Here's how the part is built. I have some questions about the finished solid (model axes, mm). Give positions to 0.01 mm unless a question says otherwise; leave off trailing zeros. Loops run counter-clockwise (first coordinate to the right, second up) from the corner with the lowest first, then second, coordinate; pieces in that order, holes last.
Q1. If we section it at C-C (x = -3): Please give me the cut outline in (y, z).
Q2. If we section it at A-A (z = 0): Please give me the cut outline in (x, y) (3 decimals), plus the area to 4 significant figures.
Q3. I need wall thicknesses on line 1 (X direction, y = 2, z = 0) (3 decimals); line 2 (X direction, y = -0.5, z = 1.75) (3 decimals); line 3 (Z direction, x = -3.5, y = 2). Which ranges of each line are inside material? Lowest first, please.
Q4. We'd pull the mould along Y, two halves only. Please class faces 1 (the face through (1, 5.969, -5)), 2 (the face through (32.51, 0.11, 0.08)), 3 (the face through (1, -5.969, -5)), 4 (the face through (1, 0, -5.969)): +Y half, -Y half, draft (parallel to the pull), parting line (faces both ways), or undercut.
Q5. If we section it at D-D (z = 4.25): Please give me the cut outline in (x, y) (3 decimals).
Q6. Will this pin go through, and if not, where does the flat tip stop? P1, Ø4.5, axis at x = -35.01, y = 0, coming from the -Z side.
Q7. If we section it at B-B (y = 1.5): Please give me the cut outline in (x, z) (3 decimals).
from build123d import *

# Parameters (mm, degrees)
F0_W     = 11.938
F0_H     = 11.938
F1_DEPTH = 40.005
F2_R     = 4.953
F3_DEPTH = 25.4
F4_R     = 4.953
F5_DEPTH = 11.939
F6_R     = 2.49936
F7_DEPTH = 11.939


with BuildPart() as f1:
    # F0 (on Right) → F1 (new body, symmetric)
    with BuildSketch(Plane.YZ):
        Rectangle(F0_W, F0_H)
    extrude(amount=F1_DEPTH, both=True)

    # F2 (on face) → F3 (cut)
    with BuildSketch(Plane.XZ.offset(5.969)):
        with Locations((3.556, 0)):
            Circle(F2_R)
    extrude(amount=-F3_DEPTH, mode=Mode.SUBTRACT)

    # F4 (on face) → F5 (cut, through all)
    with BuildSketch(Plane.XZ.offset(5.969)):
        with Locations((-3.556, 0)):
            Circle(F4_R)
    extrude(amount=-F5_DEPTH, mode=Mode.SUBTRACT)

    # F6 (on face) → F7 (cut, through all)
    with BuildSketch(Plane.XY.offset(5.969)):
        with Locations((-35.00628, 0)):
            Circle(F6_R)
        with Locations((-20.00504, 0)):
            Circle(F6_R)
        with Locations((20.00504, 0)):
            Circle(F6_R)
        with Locations((35.00628, 0)):
            Circle(F6_R)
    extrude(amount=-F7_DEPTH, mode=Mode.SUBTRACT)


solid = f1.part
Check sheet entries:
1. outline: (-5.97, -5.97) - (5.97, -5.97) - (5.97, -4.92) - (-5.97, -4.92) - close; (-5.97, 4.92) - (5.97, 4.92) - (5.97, 5.97) - (-5.97, 5.97) - close
2. outline: (-40.005, -5.969) - (-8.509, -5.969) - (-8.509, 5.969) - (-40.005, 5.969) - close; (8.509, -5.969) - (40.005, -5.969) - (40.005, 5.969) - (8.509, 5.969) - close; hole circle Ø4.999 at (-35.006, 0); hole circle Ø4.999 at (-20.005, 0); hole circle Ø4.999 at (20.005, 0); hole circle Ø4.999 at (35.006, 0)
2. area: 673.5 mm2
3. line 1: x = -40.005 to -36.505, -33.507 to -21.504, -18.506 to -8.509, 8.509 to 18.506, 21.504 to 33.507, 36.505 to 40.005
3. line 2: x = -40.005 to -37.455, -32.557 to -22.454, -17.556 to -8.19, 8.19 to 17.556, 22.454 to 32.557, 37.455 to 40.005
3. line 3: z = -5.97 to -4.95, 4.95 to 5.97
4. face 1: +Y half
4. face 2: undercut
4. face 3: -Y half
4. face 4: draft
5. outline: (-40.005, -5.969) - (-6.1, -5.969) - (-6.1, 5.969) - (-40.005, 5.969) - close; (-1.012, -5.969) - (1.012, -5.969) - (1.012, 5.969) - (-1.012, 5.969) - close; (6.1, -5.969) - (40.005, -5.969) - (40.005, 5.969) - (6.1, 5.969) - close; hole circle Ø4.999 at (-35.006, 0); hole circle Ø4.999 at (-20.005, 0); hole circle Ø4.999 at (20.005, 0); hole circle Ø4.999 at (35.006, 0)
6. P1: passes through
7. outline: (-40.005, -5.969) - (-37.005, -5.969) - (-37.005, 5.969) - (-40.005, 5.969) - close; (-33.007, -5.969) - (-22.004, -5.969) - (-22.004, 5.969) - (-33.007, 5.969) - close; (-18.006, -5.969) - (18.006, -5.969) - (18.006, 5.969) - (-18.006, 5.969) - close; (22.004, -5.969) - (33.007, -5.969) - (33.007, 5.969) - (22.004, 5.969) - close; (37.005, -5.969) - (40.005, -5.969) - (40.005, 5.969) - (37.005, 5.969) - close; hole (0, -3.448) arc R4.953 ccw (long way) to (0, 3.448) arc R4.953 ccw (long way) to start
